Can you work these out from the model? Positions are in its coordinate system, mm. A direction names the side the tool comes from. Give positions to 0.01 mm unless a question says otherwise; leave off trailing zeros. Order: outer loops, then holes, each group sorted by start corner. A loop starts at its lowest first (then second) coordinate and runs counter-clockwise, first axis right, second up. Notation, with made-up numbers: (49.5, 84.25) - (98.5, 84.25) arc R22 ccw to (98.5, 97.25) - close; hole circle Ø8 at (39.25, -11). An arc over 180 degrees is marked (long way). Return JSON: item names as keys, results as strings.
```python
from build123d import *

# Parameters (mm, degrees)
CROQUIS1_R              = 6.25
SALIENTE_EXTRUIR1_DEPTH = 1
CROQUIS2_R              = 2.45
SALIENTE_EXTRUIR2_DEPTH = 9.29
CROQUIS3_R              = 2.05
CORTAR_EXTRUIR1_DEPTH   = 14.564995393
REDONDEO1_R             = 0.5


with BuildPart() as part:
    # Croquis1 → Saliente-Extruir1 (new body)
    with BuildSketch(Plane(origin=(0, 0, 0), x_dir=(1, 0, 0), z_dir=(0, 1, 0))):
        with Locations(Location((0, 0, 0), (0, 0, 270))):
            Circle(CROQUIS1_R)
    extrude(amount=SALIENTE_EXTRUIR1_DEPTH)

    # Croquis2 → Saliente-Extruir2 (add)
    with BuildSketch(Plane(origin=(0, 1, 0), x_dir=(1, 0, 0), z_dir=(0, 1, 0))):
        with Locations(Location((0, 0, 0), (0, 0, 270))):
            Circle(CROQUIS2_R)
    extrude(amount=SALIENTE_EXTRUIR2_DEPTH)

    # Croquis3 → Cortar-Extruir1 (cut, through all)
    with BuildSketch(Plane(origin=(0, 10.29, 0), x_dir=(1, 0, 0), z_dir=(0, 1, 0))):
        with Locations(Location((0, 0, 0), (0, 0, 270))):
            Circle(CROQUIS3_R)
    extrude(amount=-CORTAR_EXTRUIR1_DEPTH, mode=Mode.SUBTRACT)

    # Redondeo1
    redondeo1_edges = [part.edges().sort_by_distance(p)[0] for p in [
        (0, 1, -2.45),
    ]]
    fillet(redondeo1_edges, radius=REDONDEO1_R)


solid = part.part
```
1. On a 3-axis mill with a long thin cutter (end or side, diameter ignored), from which of +Z, -Z, +X, -X, +Y, -Y can I reach the whole of each face in a straight line? I mean faces 4 (the face through (-3, 1, 1)), 5 (the face through (1.88, 0.49, 5.96)). Say none if no direction works.
Checks:
{"face 4": "+Y", "face 5": "+Y, -Y"}
2. Suppose I cut it at A-A (x = 0). List the corners of the cut face in (y, z) for me.
Checks:
{"outline": "(0, -6.25) - (1, -6.25) - (1, -2.95) arc R0.5 cw to (1.5, -2.45) - (10.29, -2.45) - (10.29, -2.05) - (0, -2.05) - close; (0, 2.05) - (10.29, 2.05) - (10.29, 2.45) - (1.5, 2.45) arc R0.5 cw to (1, 2.95) - (1, 6.25) - (0, 6.25) - close"}
3. For pin 1 Ø1.5 at (y, z) = (8.5, 1.5) entering from +X; pin 2 Ø4 at (y, z) = (4.5, 3.5) entering from -X; pin 3 Ø2 at (y, z) = (4.5, -1.5) entering from -X, each with a flat end and sliding along its axis, tell me the tip position at first contact or that it passes through.
Checks:
{"pin 1": "x = 2.33", "pin 2": "x = -1.94", "pin 3": "x = -2.4"}
4. If I drill on L1, parallel to X at y = 2.75, z = 0; L2, parallel to Y at x = 1, z = -4.25; L3, parallel to X at y = 1.25, z = 0.75, over which ranges is the centre line in solid material (lowest first)? Write a range as [from, to].
Checks:
{"L1": "[-2.45, -2.05], [2.05, 2.45]", "L2": "[0, 1]", "L3": "[-2.4, -1.91], [1.91, 2.4]"}
5. Suppose I cut it at B-B (z = 0). List the corners of the cut face in (x, y) for me.
Checks:
{"outline": "(-6.25, 0) - (-2.05, 0) - (-2.05, 10.29) - (-2.45, 10.29) - (-2.45, 1.5) arc R0.5 cw to (-2.95, 1) - (-6.25, 1) - close; (2.05, 0) - (6.25, 0) - (6.25, 1) - (2.95, 1) arc R0.5 cw to (2.45, 1.5) - (2.45, 10.29) - (2.05, 10.29) - close"}
6. Thinking about a two-plate mould opening in X: for faces 1 (the face through (-2, 10.29, -1)), 2 (the face through (2.033, 5.217, -0.267)), 3 (the face through (0.736, 5.833, 2.337)), which applies, +X half, -X half, draft (parallel to the pull), parting line (faces both ways), or undercut?
Checks:
{"face 1": "draft", "face 2": "undercut", "face 3": "parting line"}
7. Suppose I cut it at C-C (y = 3.5). List the corners of the cut face in (x, z) for me.
Checks:
{"outline": "circle Ø4.9 at (0, 0); hole circle Ø4.1 at (0, 0)"}
8. Suppose I cut it at D-D (x = 5). List the corners of the cut face in (y, z) for me.
Checks:
{"outline": "(0, -3.75) - (1, -3.75) - (1, 3.75) - (0, 3.75) - close"}
